The drawing under review shows one solid part. Ordinate dimensions are in mm from its lowest x, y, z. Round coordinates to 2 decimals unless told otherwise and drop trailing zeros. Order: outer loops, then holes, each group sorted by start corner. A loop starts at its lowest first (then second) coordinate and runs counter-clockwise, first axis right, second up.
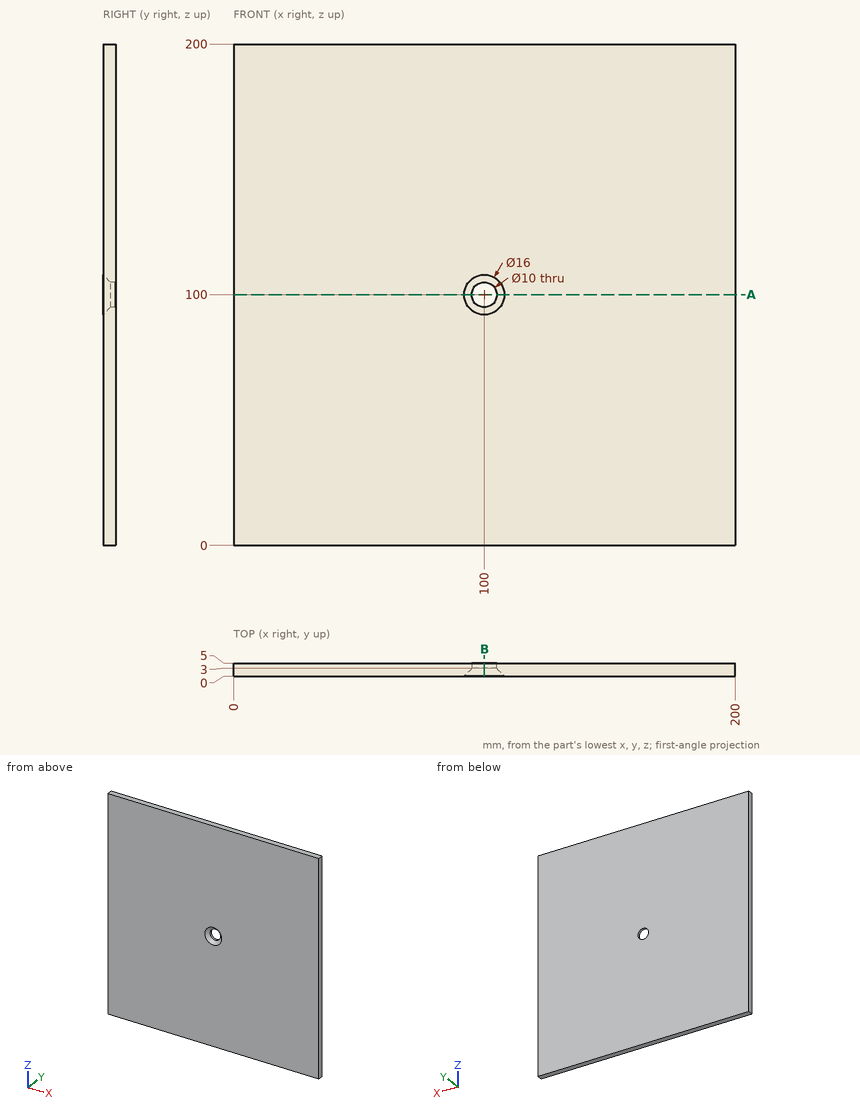
(1) We need section B-B (x = 100). Give the boundary of the cut face in (y, z), and give its area (3 significant figures).
(2) To check wall thickness, follow L1, parallel to Z at x = 100, y = 4.45; L2, parallel to Z at x = 98, y = 1.3. State the ranges of each line that lie inside material, in increasing order.
(3) We need section A-A (z = 100). Give the boundary of the cut face in (x, y), and give its area (3 significant figures).
Verdict:
1. outline: (0, 0) - (5, 0) - (5, 95) - (3, 95) - (0, 92) - close; (0, 108) - (3, 105) - (5, 105) - (5, 200) - (0, 200) - close
1. area: 941 mm2
2. L1: z = 0 to 95, 105 to 200
2. L2: z = 0 to 93.61, 106.39 to 200
3. outline: (0, 0) - (92, 0) - (95, 3) - (95, 5) - (0, 5) - close; (105, 3) - (108, 0) - (200, 0) - (200, 5) - (105, 5) - close
3. area: 941 mm2
